Model file for the job. Use its own axes, mm. Face numbers are marked on the shaded views. A direction names the side the tool comes from. Coordinates: 2 decimals unless noted, no trailing zeros. Write each loop counter-clockwise with the first axis right and the second up, starting at its lowest first coordinate (ties: lowest second). Pieces come first, ordered by that corner, then holes. Notation, with made-up numbers: (-38.5, -2) -> (-8.5, -2) arc R21 ccw to (-8.5, 19) -> close; hole circle Ø10 at (37.5, -28). An arc over 180 degrees is marked (long way). Answer as a JSON object with one key per item and string values. Group by question number.
from build123d import *

# Parameters (mm, degrees)
F1_DEPTH = 25.4


with BuildPart() as f1:
    # F0 (on Right) → F1 (new body)
    with BuildSketch(Plane.YZ):
        Polygon((-114.3, 136.525), (-215.9, 136.525), (-215.9, 34.925), (-190.5, 34.925), (-190.5, 9.525), (-139.7, 9.525), (-139.7, -73.025), (-63.5, -73.025), (-63.5, -136.525), (63.5, -136.525), (63.5, -73.025), (139.7, -73.025), (139.7, 9.525), (190.5, 9.525), (190.5, 34.925), (215.9, 34.925), (215.9, 136.525), (114.3, 136.525), (0, 85.725), align=None)
    extrude(amount=F1_DEPTH)


solid = f1.part
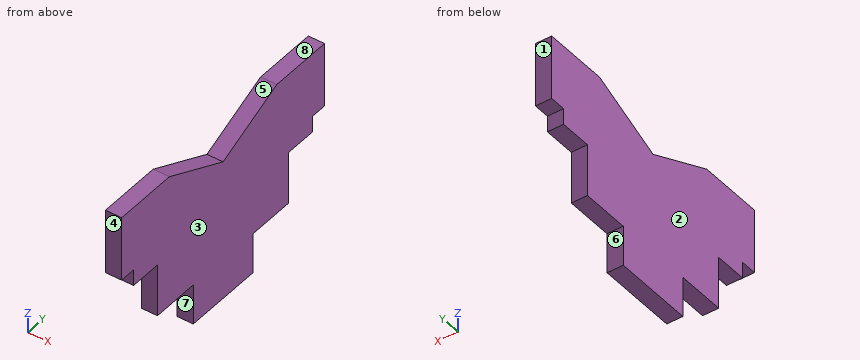
(1) Cut at A-A on x = 5.25. List the corners of the cut face in (y, z) (3 decimals), plus the area to 3 significant figures.
(2) Pull direction X, two halves, no side cores. Call the marked faces 1, 2 and 3: released by +X, released by -X, zero draft, split by the parting line, or undercut.
(3) Pin check, flat tips, straight feed: pin 1 (6 mm diameter, centred on x = 15, z = -55, fed in from -Y); pin 2 (12.5 mm diameter, centred on x = 8, y = -106.5, fed in from -Z) (3 decimals); pin 3 (7.5 mm diameter, centred on x = 10, y = -200, fed in from -Z) (3 decimals). Stop position of each tip, or through.
(4) Cut at B-B on y = -174.5. List the corners of the cut face in (x, z) (3 decimals).
(5) Cut at C-C on z = -37.5. List the corners of the cut face in (x, y).
(6) Wall check: probe 1 along Y at (x, z) = (4.25, 20); probe 2 along Y at (x, z) = (22.5, -113); probe 3 along Z at (x, y) = (11.5, 115.5) (3 decimals). Give the ranges that are in metal, low to high.
(7) 3-axis set-ups, long thin cutter, end or side, ignore diameter. For the marked faces 4, 5, 6, 7 and 8: which of +Z, -Z, +X, -X, +Y, -Y reach the whole face in a straight line?
Results found:
{
 "1": {"outline": "(-215.9, 34.925) -> (-190.5, 34.925) -> (-190.5, 9.525) -> (-139.7, 9.525) -> (-139.7, -73.025) -> (-63.5, -73.025) -> (-63.5, -136.525) -> (63.5, -136.525) -> (63.5, -73.025) -> (139.7, -73.025) -> (139.7, 9.525) -> (190.5, 9.525) -> (190.5, 34.925) -> (215.9, 34.925) -> (215.9, 136.525) -> (114.3, 136.525) -> (0, 85.725) -> (-114.3, 136.525) -> (-215.9, 136.525) -> close", "area": "78,900 mm²"},
 "2": {"face 1": "zero draft", "face 2": "released by -X", "face 3": "released by +X"},
 "3": {"pin 1": "stops at y = -139.7", "pin 2": "stops at z = -73.025", "pin 3": "stops at z = 34.925"},
 "4": {"outline": "(0, 9.525) -> (25.4, 9.525) -> (25.4, 136.525) -> (0, 136.525) -> close"},
 "5": {"outline": "(0, -139.7) -> (25.4, -139.7) -> (25.4, 139.7) -> (0, 139.7) -> close"},
 "6": {"probe 1": "y = -190.5 to 190.5", "probe 2": "y = -63.5 to 63.5", "probe 3": "z = -73.025 to 136.525"},
 "7": {"face 4": "+Z, -Z, +X, -X, -Y", "face 5": "+Z, +X, -X", "face 6": "-Z, +X, -X, +Y", "face 7": "-Z, +X, -X, -Y", "face 8": "+Z, +X, -X, +Y, -Y"}
}
